```python
from build123d import *

# Parameters (mm, degrees)
F0_W      = 660.4
F0_H      = 355.6
F1_DEPTH  = 965.2
F2_W      = 609.6
F2_H      = 914.4
F3_DEPTH  = 304.8
F4_W      = 609.6
F4_H      = 31.75
F5_DEPTH  = 304.8
F6_W      = 266.7
F6_H      = 152.4
F7_DEPTH  = 101.6
F8_W      = 25.4
F8_H      = 25.4
F9_DEPTH  = 40.64
F10_W     = 273.05
F10_H     = 215.9
F11_DEPTH = 50.8
F12_W     = 16
F12_H     = 13.3
F13_DEPTH = 19.05
F12_W_2   = 7.62
F12_H_2   = 3.81
F14_DEPTH = 0.635
F16_DEPTH = 190.5


# Not quite as in the source:
# - a feature names something its author has since deleted; it is built from what else it names


with BuildPart() as f1:
    # F0 (on Top) → F1 (new body)
    with BuildSketch(Plane.XY):
        Rectangle(F0_W, F0_H)
    extrude(amount=F1_DEPTH)

    # F2 (on face) → F3 (cut)
    with BuildSketch(Plane.XZ.offset(177.8)):
        with Locations((0, 482.6)):
            Rectangle(F2_W, F2_H)
    extrude(amount=-F3_DEPTH, mode=Mode.SUBTRACT)

    # F4 (on face) → F5 (join)
    with BuildSketch(Plane.XZ.offset(-127)):
        with Locations((0, 269.875)):
            Rectangle(F4_W, F4_H)
        with Locations((0, 428.625)):
            Rectangle(F4_W, F4_H)
    extrude(amount=F5_DEPTH)

    # F6 (on face) → F7 (join)
    with BuildSketch(Plane.XY.offset(25.4)):
        with Locations((29.1608499646, -13.5529870272)):
            Rectangle(F6_W, F6_H)
    extrude(amount=F7_DEPTH)

    # F8 (on face) → F9 (join)
    with BuildSketch(Plane.XY.offset(127)):
        with Locations((-72.4391500354, -70.7029870272)):
            Rectangle(F8_W, F8_H)
        with Locations((-72.4391500354, 43.5970129728)):
            Rectangle(F8_W, F8_H)
        with Locations((-27.9891500354, -70.7029870272)):
            Rectangle(F8_W, F8_H)
        with Locations((-27.9891500354, 43.5970129728)):
            Rectangle(F8_W, F8_H)
        with Locations((16.4608499646, -70.7029870272)):
            Rectangle(F8_W, F8_H)
        with Locations((16.4608499646, 43.5970129728)):
            Rectangle(F8_W, F8_H)
        with Locations((60.9108499646, -70.7029870272)):
            Rectangle(F8_W, F8_H)
        with Locations((60.9108499646, 43.5970129728)):
            Rectangle(F8_W, F8_H)
    extrude(amount=F9_DEPTH)

    # F10 (on face) → F11 (join)
    with BuildSketch(Plane.XY.offset(285.75)):
        Rectangle(F10_W, F10_H)
    extrude(amount=F11_DEPTH)

    # F12 (on face) → F13 (cut)
    with BuildSketch(Plane.XZ.offset(107.95)):
        with Locations((112.775, 301.9346)):
            Rectangle(F12_W, F12_H)
        with Locations((112.775, 320.375)):
            Rectangle(F12_W, F12_H)
        with Locations((93.725, 320.375)):
            Rectangle(F12_W, F12_H)
        with Locations((-33.275, 301.9346)):
            Rectangle(F12_W, F12_H)
        with Locations((93.725, 301.9346)):
            Rectangle(F12_W, F12_H)
        with Locations((-7.875, 320.375)):
            Rectangle(F12_W, F12_H)
        with Locations((-7.875, 301.9346)):
            Rectangle(F12_W, F12_H)
        with Locations((8.889, 320.375)):
            Rectangle(F12_W, F12_H)
        with Locations((8.889, 301.9346)):
            Rectangle(F12_W, F12_H)
        with Locations((25.653, 320.375)):
            Rectangle(F12_W, F12_H)
        with Locations((25.653, 301.9346)):
            Rectangle(F12_W, F12_H)
        with Locations((42.417, 320.375)):
            Rectangle(F12_W, F12_H)
        with Locations((42.417, 301.9346)):
            Rectangle(F12_W, F12_H)
        with Locations((59.181, 320.375)):
            Rectangle(F12_W, F12_H)
        with Locations((59.181, 301.9346)):
            Rectangle(F12_W, F12_H)
        with Locations((75.945, 320.375)):
            Rectangle(F12_W, F12_H)
        with Locations((75.945, 301.9346)):
            Rectangle(F12_W, F12_H)
        with Locations((-33.275, 320.375)):
            Rectangle(F12_W, F12_H)
    extrude(amount=-F13_DEPTH, mode=Mode.SUBTRACT)

    # F12 (on face) → F14 (join, symmetric)
    with BuildSketch(Plane.XZ.offset(107.95)):
        with Locations((-120.015, 295.9252057362)):
            Rectangle(F12_W_2, F12_H_2)
        with Locations((-107.315, 295.9252057362)):
            Rectangle(F12_W_2, F12_H_2)
        with Locations((-94.615, 295.9252057362)):
            Rectangle(F12_W_2, F12_H_2)
        with Locations((-81.915, 295.9252057362)):
            Rectangle(F12_W_2, F12_H_2)
        with Locations((-69.215, 295.9252057362)):
            Rectangle(F12_W_2, F12_H_2)
        with Locations((-81.915, 290.3372057362)):
            Rectangle(F12_W_2, F12_H_2)
        with Locations((-107.315, 290.3372057362)):
            Rectangle(F12_W_2, F12_H_2)
        with Locations((-69.215, 290.3372057362)):
            Rectangle(F12_W_2, F12_H_2)
        with Locations((-94.615, 290.3372057362)):
            Rectangle(F12_W_2, F12_H_2)
    extrude(amount=F14_DEPTH, both=True)

    # F15 (on face) → F16 (cut)
    with BuildSketch(Plane.XY.offset(444.5)):
        with BuildLine():
            ThreePointArc((-304.8, -63.5), (-266.7, -25.4), (-304.8, 12.7))
            Line((-304.8, 12.7), (-304.8, -63.5))
        make_face()
        with BuildLine():
            Line((304.8, -63.5), (304.8, 12.7))
            ThreePointArc((304.8, 12.7), (266.7, -25.4), (304.8, -63.5))
        make_face()
    extrude(amount=-F16_DEPTH, mode=Mode.SUBTRACT)


solid = f1.part
```
Input: part model. Units: mm. Frame: model coordinates. A direction names the side the tool comes from. Give positions to 0.01 mm unless a question says otherwise; leave off trailing zeros. Write each loop counter-clockwise with the first axis right and the second up, starting at its lowest first coordinate (ties: lowest second). Pieces come first, ordered by that corner, then holes. Notation, with made-up numbers: (59, -17) - (95, -17) arc R14 cw to (95, 10) - close; hole circle Ø3 at (-31.75, 52.5). An arc over 180 degrees is marked (long way). Write item = value, one per line. Start each with the question number.
1) Cut plane C-C (x = 231.5). Return loops of the section in (y, z), and give its area (3 significant figures).
2) Material intervals for L1, parallel to Z at x = -267.5, y = -111; L2, parallel to Z at x = 84, y = -101; L3, parallel to X at y = -82.5, z = 868, sorted ascending. Write a range as [from, to].
3) Cut plane B-B (y = -25.4). Return loops of the section in (x, z) (3 decimals).
4) Cut plane D-D (z = 270.5). Return loops of the section in (x, y), and give its area (3 significant figures).
5) Cut plane A-A (y = 97.5). Return loops of the section in (x, z) (3 decimals), and give its area (3 significant figures).
6) Pin query (flat end, axial travel): pin 1 (10.5 mm diameter, centred on x = 27.5, z = 317.5, fed in from -Y); pin 2 (2 mm diameter, centred on x = 207, z = 515, fed in from -Y); pin 3 (7.5 mm diameter, centred on x = 64.5, z = 154, fed in from -Y). Return the tip coordinate at first contact, or that it passes through.
7) Reachability of faces 1 (the face through (61, 56.297, 147)), 2 (the face through (-4, -23, 444.5)) from +Z, -Z, +X, -X, +Y, -Y: full face, straight path, thin tool, end or side. Return the list, or none.
Answers follow:
q1.outline = (-177.8, 0) - (177.8, 0) - (177.8, 965.2) - (-177.8, 965.2) - (-177.8, 939.8) - (127, 939.8) - (127, 444.5) - (-177.8, 444.5) - (-177.8, 412.75) - (127, 412.75) - (127, 285.75) - (-177.8, 285.75) - (-177.8, 254) - (127, 254) - (127, 25.4) - (-177.8, 25.4) - close
q1.area = 83,900 mm^2
q2.L1 = [0, 25.4], [254, 285.75], [412.75, 444.5], [939.8, 965.2]
q2.L2 = [0, 25.4], [254, 336.55], [412.75, 444.5], [939.8, 965.2]
q2.L3 = [-330.2, -304.8], [304.8, 330.2]
q3.outline = (-330.2, 0) - (330.2, 0) - (330.2, 965.2) - (-330.2, 965.2) - close; (-266.7, 254) - (266.7, 254) - (266.7, 285.75) - (136.525, 285.75) - (136.525, 336.55) - (-136.525, 336.55) - (-136.525, 285.75) - (-266.7, 285.75) - close; (-266.7, 412.75) - (266.7, 412.75) - (266.7, 444.5) - (-266.7, 444.5) - close; hole (-304.8, 25.4) - (-104.189, 25.4) - (-104.189, 127) - (162.511, 127) - (162.511, 25.4) - (304.8, 25.4) - (304.8, 939.8) - (-304.8, 939.8) - close
q4.outline = (-330.2, -177.8) - (330.2, -177.8) - (330.2, 177.8) - (-330.2, 177.8) - close; hole (-304.8, -63.5) arc R38.1 ccw to (-304.8, 12.7) - close; hole (304.8, -63.5) - (304.8, 12.7) arc R38.1 ccw to start
q4.area = 230,000 mm^2
q5.outline = (-330.2, 0) - (330.2, 0) - (330.2, 965.2) - (-330.2, 965.2) - close; hole (-304.8, 25.4) - (304.8, 25.4) - (304.8, 254) - (-304.8, 254) - close; hole (-304.8, 285.75) - (-136.525, 285.75) - (-136.525, 336.55) - (136.525, 336.55) - (136.525, 285.75) - (304.8, 285.75) - (304.8, 412.75) - (-304.8, 412.75) - close; hole (-304.8, 444.5) - (304.8, 444.5) - (304.8, 939.8) - (-304.8, 939.8) - close
q5.area = 133,000 mm^2
q6.pin_1 = -107.95
q6.pin_2 = 127
q6.pin_3 = -83.4
q7.face_1 = none
q7.face_2 = -Y
